from build123d import *

# Parameters (mm, degrees)
IZIM1_W                     = 105
IZIM1_H                     = 61
IZIM1_W_2                   = 99
IZIM1_H_2                   = 40
Y_KSEKLIK_EKSTR_ZYON1_DEPTH = 11
IZIM2_W                     = 113
IZIM2_H                     = 69
IZIM2_W_2                   = 105
IZIM2_H_2                   = 61
Y_KSEKLIK_EKSTR_ZYON2_DEPTH = 70
IZIM3_W                     = 113
IZIM3_H                     = 69
IZIM3_W_2                   = 99
IZIM3_H_2                   = 40
Y_KSEKLIK_EKSTR_ZYON3_DEPTH = 1
IZIM4_R                     = 24.5
KES_EKSTR_ZYON1_DEPTH       = 7
IZIM5_R                     = 3
KES_EKSTR_ZYON2_DEPTH       = 7
IZIM6_R                     = 5.666240849
IZIM6_W                     = 11
IZIM6_H                     = 10
KES_EKSTR_ZYON3_DEPTH       = 7
RADYUS1_R                   = 4
RADYUS2_R                   = 3
RADYUS4_R                   = 8
IZIM14_W                    = 105
IZIM14_H                    = 61
Y_KSEKLIK_EKSTR_ZYON8_DEPTH = 5


# Some blends are built 0.0001 mm under size
with BuildPart() as part:
    # izim1 → Y_kseklik-Ekstr_zyon1 (new body)
    with BuildSketch(Plane.XY):
        Rectangle(IZIM1_W, IZIM1_H)
        Rectangle(IZIM1_W_2, IZIM1_H_2, mode=Mode.SUBTRACT)
    extrude(amount=Y_KSEKLIK_EKSTR_ZYON1_DEPTH)



with BuildPart() as body_2:
    # izim2 → Y_kseklik-Ekstr_zyon2 (new body)
    with BuildSketch(Plane(origin=(0, 0, 0), x_dir=(-1, 0, 0), z_dir=(0, 0, -1))):
        Rectangle(IZIM2_W, IZIM2_H)
        Rectangle(IZIM2_W_2, IZIM2_H_2, mode=Mode.SUBTRACT)
    extrude(amount=Y_KSEKLIK_EKSTR_ZYON2_DEPTH)


with BuildPart() as part_1:
    add(part.part)

    add(body_2.part)  # Y_kseklik-Ekstr_zyon3 merges body 2
    # izim3 → Y_kseklik-Ekstr_zyon3 (add)
    with BuildSketch(Plane.XY):
        Rectangle(IZIM3_W, IZIM3_H)
        Rectangle(IZIM3_W_2, IZIM3_H_2, mode=Mode.SUBTRACT)
    extrude(amount=Y_KSEKLIK_EKSTR_ZYON3_DEPTH)

    # izim4 → Kes-Ekstr_zyon1 (cut)
    with BuildSketch(Plane.ZY.offset(56.5)):
        with Locations((-24, 0)):
            Circle(IZIM4_R)
    extrude(amount=-KES_EKSTR_ZYON1_DEPTH, mode=Mode.SUBTRACT)

    # izim5 → Kes-Ekstr_zyon2 (cut)
    with BuildSketch(Plane(origin=(0, 34.5, 0), x_dir=(1, 0, 0), z_dir=(0, 1, 0))):
        with Locations(Location((12, 45, 0), (0, 0, 270))):
            Circle(IZIM5_R)
    extrude(amount=-KES_EKSTR_ZYON2_DEPTH, mode=Mode.SUBTRACT)

    # izim6 → Kes-Ekstr_zyon3 (cut)
    with BuildSketch(Plane(origin=(0, -34.5, 0), x_dir=(-1, 0, 0), z_dir=(0, -1, 0))):
        with Locations(Location((41.5, 19, 0), (0, 0, 90))):
            Circle(IZIM6_R)
        with Locations(Location((21.5, 19, 0), (0, 0, 90))):
            Circle(IZIM6_R)
        with Locations((-44, 20)):
            Rectangle(IZIM6_W, IZIM6_H)
    extrude(amount=-KES_EKSTR_ZYON3_DEPTH, mode=Mode.SUBTRACT)

    # Radyus1
    radyus1_edges = [part_1.edges().sort_by_distance(p)[0] for p in [
        (0, -30.5, 1),
        (52.5, 0, 1),
        (0, 30.5, 1),
        (-52.5, 0, 1),
    ]]
    fillet(radyus1_edges, radius=RADYUS1_R - 0.0001)  # a hair under: the kernel refuses the full size

    # Radyus2
    radyus2_edges = [part_1.edges().sort_by_distance(p)[0] for p in [
        (-52.5, 0, 11),
        (0, -30.5, 11),
        (52.5, 0, 11),
        (0, 30.5, 11),
    ]]
    fillet(radyus2_edges, radius=RADYUS2_R - 0.0001)  # a hair under: the kernel refuses the full size

    # Radyus4
    # the kernel refuses this fillet: 8 mm, written as the material it takes off along each edge
    with BuildSketch(Plane(origin=(56.5, -34.5, 21), x_dir=(0, 1, 0), z_dir=(0, 0, -1)), Plane(origin=(56.5, 34.5, 21), x_dir=(-1, 0, 0), z_dir=(0, 0, -1)), Plane(origin=(-56.5, 34.5, -90), x_dir=(1, 0, 0), z_dir=(0, 0, 1))) as radyus4_piece_1:
        with BuildLine():
            CenterArc((RADYUS4_R, -RADYUS4_R), RADYUS4_R, 90, 90)
            Line((0, -RADYUS4_R), (0, 0))
            Line((0, 0), (RADYUS4_R, 0))
        make_face()
    extrude(amount=111, mode=Mode.SUBTRACT)
    with BuildSketch(Plane(origin=(-56.5, -34.5, 21), x_dir=(0, 1, 0), z_dir=(0, 0, -1))) as radyus4_piece_2:
        with BuildLine():
            CenterArc((RADYUS4_R, RADYUS4_R), RADYUS4_R, 180, 90)
            Line((0, RADYUS4_R), (0, 0))
            Line((0, 0), (RADYUS4_R, 0))
        make_face()
    extrude(amount=111, mode=Mode.SUBTRACT)

    # izim14 → Y_kseklik-Ekstr_zyon8 (add)
    with BuildSketch(Plane(origin=(0, 0, -70), x_dir=(-1, 0, 0), z_dir=(0, 0, -1))):
        with BuildLine():
            Line((-56.5, 26.5), (-56.5, -26.5))
            ThreePointArc((-56.5, -26.5), (-54.156854249, -32.156854249), (-48.5, -34.5))
            Line((-48.5, -34.5), (48.5, -34.5))
            ThreePointArc((48.5, -34.5), (54.156854249, -32.156854249), (56.5, -26.5))
            Line((56.5, -26.5), (56.5, 26.5))
            ThreePointArc((56.5, 26.5), (54.156854249, 32.156854249), (48.5, 34.5))
            Line((48.5, 34.5), (-48.5, 34.5))
            ThreePointArc((-48.5, 34.5), (-54.156854249, 32.156854249), (-56.5, 26.5))
        make_face()
        Rectangle(IZIM14_W, IZIM14_H, mode=Mode.SUBTRACT)
    extrude(amount=Y_KSEKLIK_EKSTR_ZYON8_DEPTH)


solid = part_1.part
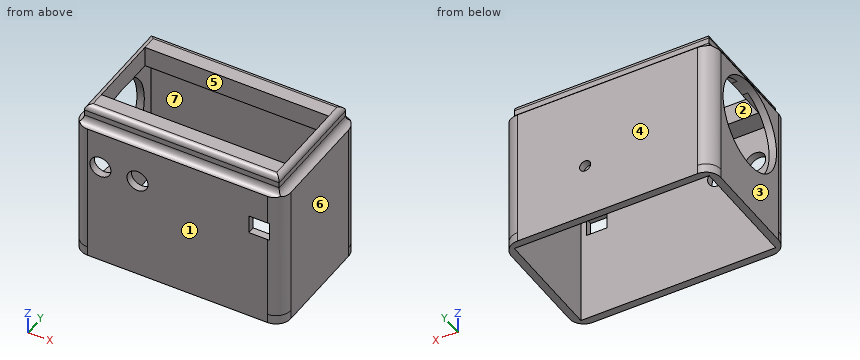
Read the model definition and answer for the solid it produces. Units are mm, in the model's axes. Face numbers are marked on the shaded views. A direction names the side the tool comes from. Coordinates: 2 decimals unless noted, no trailing zeros. Write each loop counter-clockwise with the first axis right and the second up, starting at its lowest first coordinate (ties: lowest second). Pieces come first, ordered by that corner, then holes. Notation, with made-up numbers: M -6,68.25 L 7,68.25 A19 ccw 7,80.25 Z; hole C 54,78 d3. An arc over 180 degrees is marked long. Use a Markdown table: item, result.
Q1. The part is cut by section C-C, the plane z = -59. Write down the section's boundary in (x, y).
Answer block:
| item | result |
|---|---|
| outline | M -56.5,-26.5 A8 ccw -48.5,-34.5 L 48.5,-34.5 A8 ccw 56.5,-26.5 L 56.5,26.5 A8 ccw 48.5,34.5 L -48.5,34.5 A8 ccw -56.5,26.5 Z; hole M -52.5,-30.5 L 52.5,-30.5 L 52.5,30.5 L -52.5,30.5 Z |
Q2. Determine the mould class of the marked faces 1, 2, 3 and 4 for opening direction Y: released by +Y, released by -Y, zero draft, split by the parting line, or undercut.
Answer block:
| item | result |
|---|---|
| face 1 | released by -Y |
| face 2 | undercut |
| face 3 | zero draft |
| face 4 | released by +Y |
Q3. Which of the six approach directions +Z, -Z, +X, -X, +Y, -Y give full straight-line access (tool end or side, diameter ignored) to the marked faces 5, 6 and 7?
Answer block:
| item | result |
|---|---|
| face 5 | +Z, -Z |
| face 6 | +Z, -Z, +X, +Y, -Y |
| face 7 | -Z |
Q4. Straight lines are drawn through the part: L1, parallel to Y at x = -28, z = -63.5; L2, parallel to X at y = -3, z = -62; L3, parallel to X at y = -33.5, z = -19. For each, find the intervals that lie inside material, in ascending order. Write a range as [from, to].
Answer block:
| item | result |
|---|---|
| L1 | y = [-34.5, -30.5], [30.5, 34.5] |
| L2 | x = [-56.5, -52.5], [52.5, 56.5] |
| L3 | x = [-52.37, -47.17], [-35.83, -27.17], [-15.83, 38.5], [49.5, 52.37] |
Q5. The part is cut by section A-A, the plane y = 0. Give the number of separate pieces and of enclosed holes in the cut face, then the cut area to 3 significant figures.
Answer block:
| item | result |
|---|---|
| separate pieces | 3 |
| enclosed holes | 0 |
| area | 480 mm2 |
Q6. Each of these flat-tipped pins is pushed along its axis until it touches: pin 1 Ø1.2 at (y, z) = (-31.5, -21.5) entering from +X; pin 2 Ø2.5 at (y, z) = (-8.5, 6.5) entering from +X; pin 3 Ø2 at (x, y) = (46.5, -32) entering from +Z. Where does it stop, or does it pass through?
Answer block:
| item | result |
|---|---|
| pin 1 | stops at x = 55.18 |
| pin 2 | stops at x = 52.5 |
| pin 3 | stops at z = 3.06 |
